from build123d import *

# Parameters (mm, degrees)
BOSS_EXTRUDE2_DEPTH = 25
SKETCH6_R           = 1.25
CUT_EXTRUDE1_DEPTH  = 65.847898964


with BuildPart() as part:
    # Sketch3 → Boss-Extrude2 (new body)
    with BuildSketch(Plane(origin=(0, 0, 0), x_dir=(1, 0, 0), z_dir=(0, 1, 0))):
        Polygon((0, 18.25), (0, 22.25), (38.64701272, 22.25), (40, 20.89701272), (40, -20.89701272), (38.64701272, -22.25), (0, -22.25), (0, -18.25), (34.64701272, -18.25), (36, -16.89701272), (36, 16.89701272), (34.64701272, 18.25), align=None)
    extrude(amount=BOSS_EXTRUDE2_DEPTH)

    # Sketch6 → Cut-Extrude1 (cut, through all)
    with BuildSketch(Plane.XY.offset(22.25)):
        with Locations((10, 12.5)):
            Circle(SKETCH6_R)
    extrude(amount=-CUT_EXTRUDE1_DEPTH, mode=Mode.SUBTRACT)


solid = part.part
Design review of the part built by this model. Coordinates are the model's own, in mm. A direction names the side the tool comes from. Give positions to 0.01 mm unless a question says otherwise; leave off trailing zeros. Loops run counter-clockwise (first coordinate to the right, second up) from the corner with the lowest first, then second, coordinate; pieces in that order, holes last. Notation, with made-up numbers: (2.25, 22.25) - (20.25, 22.25) arc R14 ccw to (20.25, 47.25) - close; hole circle Ø9 at (-26, 5.5). An arc over 180 degrees is marked (long way). Write item = value, one per line.
1) Take a section at D-D on z = -16. State the section outline as (x, y) points.
Result sheet:
outline = (36, 0) - (40, 0) - (40, 25) - (36, 25) - close
2) Tool access review of faces 1 (the face through (9.079, 13.345, -20.222)), 2 (the face through (17, 12, 18.25)): name each direction out of +Z, -Z, +X, -X, +Y, -Y from which nothing blocks a thin tool from reaching the whole face with its end or side.
Result sheet:
face_1 = +Z, -Z
face_2 = -X, +Y, -Y
3) Take a section at A-A on y = 12.5. State the section outline as (x, z) points, and give its area (3 significant figures).
Result sheet:
outline = (0, -22.25) - (8.75, -22.25) - (8.75, -18.25) - (0, -18.25) - close; (0, 18.25) - (8.75, 18.25) - (8.75, 22.25) - (0, 22.25) - close; (11.25, -22.25) - (38.65, -22.25) - (40, -20.9) - (40, 20.9) - (38.65, 22.25) - (11.25, 22.25) - (11.25, 18.25) - (34.65, 18.25) - (36, 16.9) - (36, -16.9) - (34.65, -18.25) - (11.25, -18.25) - close
area = 446 mm2
4) To check wall thickness, follow line 1 (Y direction, x = 10, z = -20); line 2 (Z direction, x = 23, y = 21); line 3 (X direction, y = 22, z = -10). State the ranges of each line that lie inside material, in increasing order.
Result sheet:
line_1 = 0 to 11.25, 13.75 to 25
line_2 = -22.25 to -18.25, 18.25 to 22.25
line_3 = 36 to 40
5) Take a section at C-C on y = 21.75. State the section outline as (x, z) points.
Result sheet:
outline = (0, -22.25) - (38.65, -22.25) - (40, -20.9) - (40, 20.9) - (38.65, 22.25) - (0, 22.25) - (0, 18.25) - (34.65, 18.25) - (36, 16.9) - (36, -16.9) - (34.65, -18.25) - (0, -18.25) - close
6) Clearance check with flat-ended pins moving along their axes: pin 1 Ø6 at (x, z) = (8.5, -15.5) entering from +Y; pin 2 Ø12 at (y, z) = (15.5, 5.5) entering from -X. State where each tip first meets the part, or that it passes through.
Result sheet:
pin_1 = 25
pin_2 = 36
7) Take a section at B-B on x = 10. State the section outline as (y, z) points, and give its area (3 significant figures).
Result sheet:
outline = (0, -22.25) - (11.25, -22.25) - (11.25, -18.25) - (0, -18.25) - close; (0, 18.25) - (11.25, 18.25) - (11.25, 22.25) - (0, 22.25) - close; (13.75, -22.25) - (25, -22.25) - (25, -18.25) - (13.75, -18.25) - close; (13.75, 18.25) - (25, 18.25) - (25, 22.25) - (13.75, 22.25) - close
area = 180 mm2
8) Draft analysis for pull direction Z (two halves, no side actions). For faces 3 (the face through (18, 12, -18.25)), 4 (the face through (20, 12, 22.25)), 5 (the face through (0, 12, -20)), state which applies: +Z half, -Z half, draft (parallel to the pull), parting line (faces both ways), or undercut.
Result sheet:
face_3 = undercut
face_4 = +Z half
face_5 = draft
